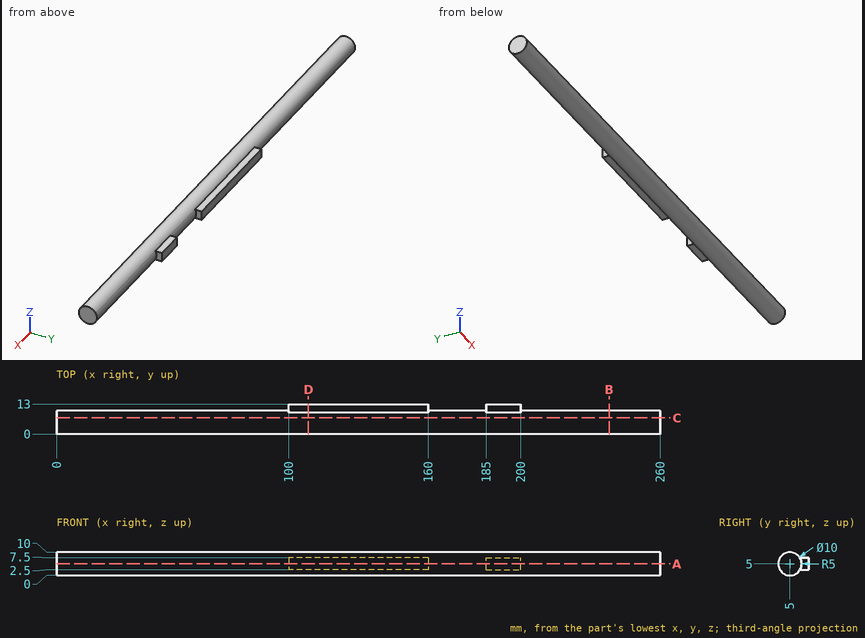
Can you work these out from the drawing? Everything is in mm from the part's minimum corner. Give positions to 0.01 mm unless a question says otherwise; leave off trailing zeros. Order: outer loops, then holes, each group sorted by start corner. A loop starts at its lowest first (then second) coordinate and runs counter-clockwise, first axis right, second up.
Item 1: I'm going to push flat-ended pins straight in: pin 1 (1.5 mm diameter, centred on x = 161, y = 2, fed in from -Z); pin 2 (1.8 mm diameter, centred on x = 195.5, y = 11, fed in from +Z); pin 3 (1.1 mm diameter, centred on x = 193, y = 10.5, fed in from -Z); pin 4 (4 mm diameter, centred on y = 11, z = 5, fed in from -X). Where does each tip first touch, or does it pass through?
Item 2: If we section it at C-C, the plane y = 7: Write out the boundary of the cut face in (x, z), plus the area to 3 significant figures.
Item 3: If we section it at B-B, the plane x = 238: Write out the boundary of the cut face in (y, z), plus the area to 3 significant figures.
Item 4: I need wall thicknesses on line 1 (X direction, y = 11.25, z = 3); line 2 (Z direction, x = 105, y = 4.5); line 3 (Z direction, x = 109, y = 3.5). Which ranges of each line are inside material? Lowest first, please.
Item 5: If we section it at D-D, the plane x = 108.5: Write out the boundary of the cut face in (y, z).
Item 6: If we section it at A-A, the plane z = 5: Write out the boundary of the cut face in (x, y).
Values:
1. pin 1: stops at z = 0.53
1. pin 2: stops at z = 7.5
1. pin 3: stops at z = 2.5
1. pin 4: stops at x = 0
2. outline: (0, 0.42) - (260, 0.42) - (260, 9.58) - (0, 9.58) - close
2. area: 2,380 mm2
3. outline: circle Ø10 at (5, 5)
3. area: 78.5 mm2
4. line 1: x = 100 to 160, 185 to 200
4. line 2: z = 0.03 to 9.97
4. line 3: z = 0.23 to 9.77
5. outline: (9.33, 2.5) - (13, 2.5) - (13, 7.5) - (9.33, 7.5) arc R5 ccw (long way) to start
6. outline: (0, 0) - (260, 0) - (260, 10) - (200, 10) - (200, 13) - (185, 13) - (185, 10) - (160, 10) - (160, 13) - (100, 13) - (100, 10) - (0, 10) - close
